Autodesk Inventor part; units mm, degrees
ref_plane "YZ Plane" through (0, 0, 0) normal (1, 0, 0) x (0, 1, 0)
ref_plane "XZ Plane" through (0, 0, 0) normal (0, 1, 0) x (-1, 0, 0)
ref_plane "XY Plane" through (0, 0, 0) normal (0, 0, 1) x (1, 0, 0)
sketch "Sketch1" plane through (0, 0, 0) normal (0, 0, 1) x (1, 0, 0)
  circle A0 centre (0, 0) radius 23.965
  circle A1 centre (0, 0) radius 30
  spline S0 degree 3 poles (-14.0044, 16.3473) (-10.6248, 19.2425) (-6.3279, 21.0504) (-1.895, 21.4422) (2.5312, 21.8334) (7.0716, 20.8109) (10.9029, 18.5603) (14.7508, 16.3) (17.8645, 12.8114) (19.6749, 8.7325) (21.4787, 4.6683) (21.9802, 0.0378) (21.0881, -4.3184) (20.1947, -8.6815) (17.9074, -12.7482) (14.643, -15.7779) (13.057, -17.2497) (11.2477, -18.4805) (9.2962, -19.4149) knots 101.316363 101.316363 101.316363 101.316363 101.936571 101.936571 101.936571 102.555845 102.555845 102.555845 103.177798 103.177798 103.177798 103.797501 103.797501 103.797501 104.418203 104.418203 104.418203 104.719755 104.719755 104.719755 104.719755 construction
  circle A2 centre (0, 0) radius 20.7257 construction
  line L0 (9.2962, -19.4149) -> (0, 0) construction
  dimension "d0" = 47.93
  dimension "d2" = 60
  dimension "d26" = 6.035
  dimension "d27" = 21.5257
extrude "Extrusion1" add sketch "Sketch1" along normal blind 25
sketch "Sketch3" plane through (0, 0, 25) normal (0, 0, 1) x (1, 0, 0)
  circle A0 centre (0, 0) radius 23.965 construction
  circle A1 centre (0, 0) radius 30
  circle A2 centre (0, 0) radius 18
  dimension "d25" = 36
extrude "Extrusion2" add sketch "Sketch3" along normal blind 10
chamfer "Chamfer2" distance 2 angle 45 2 edges at (-30, 0, 35) (-18, 0, 35)
thread "Thread2"
equation "\"d0\" = Tread_OD"
equation "\"d2\" = NutCap_OD"
equation "\"d3\" = NutCapTread_L"
equation "\"d25\" = Screw_DIA"
equation "\"TD\" = 0.3"
equation "\"Ball_DIA\" = 6"
equation "\"Screw_L\" = 292"
equation "\"Screw_DIA\" = 36"
equation "\"Nut_OD\" = 66"
equation "\"BPath_REVQ\" = 5.75"
equation "\"Tread_OFFSET\" = 8.075"
equation "\"SteeringColumn_DIA\" = 26"
equation "\"SteeringColumnChamfer_DEG\" = 20deg"
equation "\"Rack_L\" = 307.252"
equation "\"NutCapTread_L\" = 25"
equation "\"NutCapTread_THICKNESS\" = 5.365"
equation "\"NutCap_OD\" = 60"
equation "\"SupportFlange_THICKNESS\" = 5"
equation "\"GearKey_L\" = 32"
properties part number "MCEN4000:B4" material "STAINLESS STEEL, AISI 302"
Design review of the part built by this model. Coordinates are the model's own, in mm. A direction names the side the tool comes from. Coordinates: 2 decimals unless noted, no trailing zeros. Write each loop counter-clockwise with the first axis right and the second up, starting at its lowest first coordinate (ties: lowest second). Pieces come first, ordered by that corner, then holes. Notation, with made-up numbers: (78, 31.25) - (122, 31.25) arc R21 ccw to (122, 61.25) - close; hole circle Ø8 at (-8, -10). An arc over 180 degrees is marked (long way). One line per item, written item: value.
1) Add section D-D (z = 31.5). State the section outline as (x, y) points, plus the area to 3 significant figures.
Answer sheet:
outline: circle Ø60 at (0, 0); hole circle Ø36 at (0, 0)
area: 1,810 mm2
2) Add section A-A (x = 0). State the section outline as (y, z) points (3 decimals), plus the area to 3 significant figures.
Answer sheet:
outline: (-30, 0) - (-23.965, 0) - (-23.965, 25) - (-18, 25) - (-18, 33) - (-20, 35) - (-28, 35) - (-30, 33) - close; (18, 25) - (23.965, 25) - (23.965, 0) - (30, 0) - (30, 33) - (28, 35) - (20, 35) - (18, 33) - close
area: 534 mm2
3) To check wall thickness, follow probe 1 along Y at (x, z) = (0, 14) (3 decimals); probe 2 along Y at (x, z) = (0, 31); probe 3 along X at (y, z) = (-8.5, 12). State the ranges of each line that lie inside material, in increasing order.
Answer sheet:
probe 1: y = -30 to -23.965, 23.965 to 30
probe 2: y = -30 to -18, 18 to 30
probe 3: x = -28.77 to -22.41, 22.41 to 28.77
4) Add section C-C (z = 14). State the section outline as (x, y) points (3 decimals).
Answer sheet:
outline: circle Ø60 at (0, 0); hole circle Ø47.93 at (0, 0)
5) Insertion check: pin 1 (4 mm diameter, centred on x = 17.5, z = 26.5, fed in from +Y); pin 2 (8 mm diameter, centred on y = -24, z = 26.5, fed in from +X); pin 3 (2 mm diameter, centred on x = -6, z = 7, fed in from +Y). Each pin has a flat end and moves straight along its axis. Give the tip position at first contact, or say it passes through.
Answer sheet:
pin 1: stops at y = 25.69
pin 2: stops at x = 22.36
pin 3: stops at y = 29.58
6) For faces 1 (the face through (-6.1, 27.46, 34.87)), 2 (the face through (3, 18, 25)), list the 3-axis set-ups (+Z, -Z, +X, -X, +Y, -Y) from which the entire face can be reached by the end or side of a thin tool; tool diameter is ignored.
Answer sheet:
face 1: +Z
face 2: -Z
7) Mouldability with a two-part tool opening along Y and no side actions: class faces 3 (the face through (-7, 19, 35)), 4 (the face through (-29.97, -1.32, 16.27)), 5 (the face through (-2.343, -17.847, 28.944)), 6 (the face through (-3.929, -17.694, 33.125)) as +Y half, -Y half, draft (parallel to the pull), parting line (faces both ways), or undercut.
Answer sheet:
face 3: draft
face 4: parting line
face 5: undercut
face 6: undercut
